Work out the finished part from the listing and answer in its coordinate system (mm). A direction names the side the tool comes from. Give positions to 0.01 mm unless a question says otherwise; leave off trailing zeros. Order: outer loops, then holes, each group sorted by start corner. A loop starts at its lowest first (then second) coordinate and runs counter-clockwise, first axis right, second up. Notation, with made-up numbers: M -21.5,41.5 L -17.5,41.5 A26 cw -17.5,60.5 Z; hole C 76,-36.5 d11. An arc over 180 degrees is marked long. One line per item, written item: value.
from build123d import *

# Parameters (mm, degrees)
SKETCH_1_W      = 19
SKETCH_1_H      = 15.2
EXTRUDE_1_DEPTH = 15
SKETCH_2_W      = 1
SKETCH_2_H      = 1
EXTRUDE_2_DEPTH = 3.5


with BuildPart() as part:
    # 草图1 → 拉伸1 (new body)
    with BuildSketch(Plane(origin=(0, 0, 0), x_dir=(1, 0, 0), z_dir=(0, 1, 0))):
        Rectangle(SKETCH_1_W, SKETCH_1_H)
    extrude(amount=EXTRUDE_1_DEPTH)

    # 草图2 → 拉伸2 (add)
    with BuildSketch(Plane.XZ):
        with Locations((8.23, 0)):
            Rectangle(SKETCH_2_W, SKETCH_2_H)
        with Locations((5.77, 6.33)):
            Rectangle(SKETCH_2_W, SKETCH_2_H)
        with Locations((-6.96, 6.33)):
            Rectangle(SKETCH_2_W, SKETCH_2_H)
        with Locations((-6.96, -6.33)):
            Rectangle(SKETCH_2_W, SKETCH_2_H)
        with Locations((5.77, -6.33)):
            Rectangle(SKETCH_2_W, SKETCH_2_H)
    extrude(amount=EXTRUDE_2_DEPTH)


solid = part.part
(1) Find the intervals of material crossed by probe 1 along Y at (x, z) = (7.25, -1.25); probe 2 along X at (y, z) = (-1.5, 0), in increasing order. Write a range as from..to.
Findings:
probe 1: y = 0..15
probe 2: x = 7.73..8.73
(2) Section B-B, the plane x = -7 is taken. Give the vertices of the cut face in (y, z).
Findings:
outline: M -3.5,-6.83 L 0,-6.83 L 0,-7.6 L 15,-7.6 L 15,7.6 L 0,7.6 L 0,6.83 L -3.5,6.83 L -3.5,5.83 L 0,5.83 L 0,-5.83 L -3.5,-5.83 Z
(3) Determine the mould class of faces 1 (the flat face through (5.27, -2, -6)), 2 (the flat face through (-7, -2, 6.83)), 3 (the flat face through (6, -2, 5.83)) for opening direction Z: pulls with the +Z half, pulls with the -Z half, needs draft (parallel to the pull), parting line crosses it, or undercut.
Findings:
face 1: needs draft
face 2: pulls with the +Z half
face 3: undercut
(4) Section D-D, the plane z = 3.75 is taken. Give the vertices of the cut face in (x, y).
Findings:
outline: M -9.5,0 L 9.5,0 L 9.5,15 L -9.5,15 Z
(5) Given P1, Ø0.8, axis at y = -1.5, z = -6, coming from the -X side; P2, Ø1.1, axis at x = 5.5, y = -2, coming from the +Z side; P3, Ø0.5, axis at y = -1.5, z = 6, coming from the +X side, each flat-ended and moving along its own axis, determine where each tip first touches the part or whether it passes through.
Findings:
P1: stops at x = -7.46
P2: stops at z = 6.83
P3: stops at x = 6.27
(6) Section C-C, the plane z = -6.5 is taken. Give the vertices of the cut face in (x, y), then the cut area to 3 significant figures.
Findings:
outline: M -9.5,0 L -7.46,0 L -7.46,-3.5 L -6.46,-3.5 L -6.46,0 L 5.27,0 L 5.27,-3.5 L 6.27,-3.5 L 6.27,0 L 9.5,0 L 9.5,15 L -9.5,15 Z
area: 292 mm^2
(7) Which of the six approach directions +Z, -Z, +X, -X, +Y, -Y give full straight-line access (tool end or side, diameter ignored) to faces 4 (the flat face through (-7, -2, 5.83)), 5 (the flat face through (-7.46, -2, -6)), 6 (the flat face through (-7, -2, -6.83)), 7 (the flat face through (-6.46, -2, -6)), 8 (the flat face through (6, -2, 6.83))?
Findings:
face 4: +X, -X, -Y
face 5: +Z, -Z, -X, -Y
face 6: -Z, +X, -X, -Y
face 7: +Z, -Z, -Y
face 8: +Z, +X, -X, -Y
(8) Section A-A, the plane y = -0.25 is taken. Give the vertices of the cut face in (x, z), then the cut area to 3 significant figures.
Findings:
outline: M -7.46,-6.83 L -6.46,-6.83 L -6.46,-5.83 L -7.46,-5.83 Z; M -7.46,5.83 L -6.46,5.83 L -6.46,6.83 L -7.46,6.83 Z; M 5.27,-6.83 L 6.27,-6.83 L 6.27,-5.83 L 5.27,-5.83 Z; M 5.27,5.83 L 6.27,5.83 L 6.27,6.83 L 5.27,6.83 Z; M 7.73,-0.5 L 8.73,-0.5 L 8.73,0.5 L 7.73,0.5 Z
area: 5.00 mm^2
